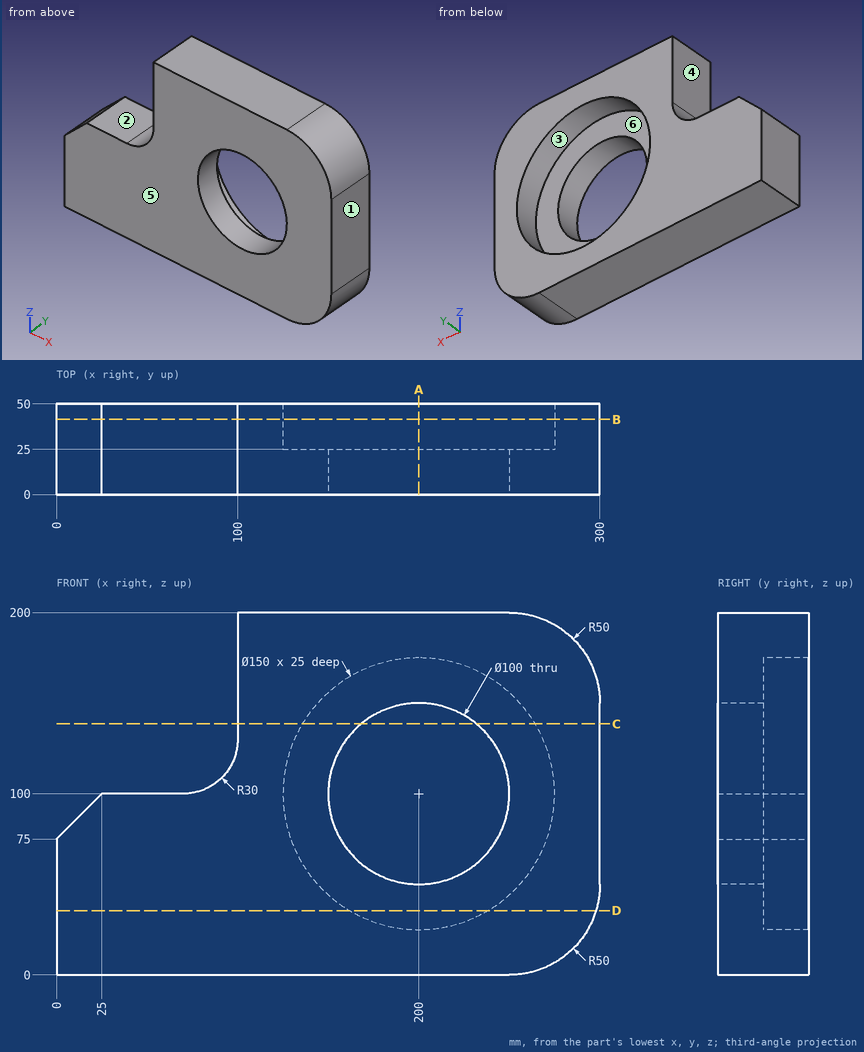
Geometry check sheet. Reference: drawing and pictorial views, mm from the part's lowest x, y, z. A direction names the side the tool comes from. Round coordinates to 2 decimals unless told otherwise and drop trailing zeros. Loops run counter-clockwise (first coordinate to the right, second up) from the corner with the lowest first, then second, coordinate; pieces in that order, holes last. Notation, with made-up numbers: (79.25, 43) -> (122.25, 43) arc R25 cw to (122.25, 80) -> close; hole circle Ø3 at (40, -6.75). An arc over 180 degrees is marked (long way). Answer as a JSON object with one key per item and string values.
Q1. Scan lines: line 1 (Z direction, x = 200, y = 16.25); line 2 (Z direction, x = 200, y = 35.25); line 3 (Y direction, x = 196, z = 32). Record each from-to range of solid material in increasing order. Write a range as from..to.
Data:
{"line 1": "z = 0..50, 150..200", "line 2": "z = 0..25, 175..200", "line 3": "y = 0..25"}
Q2. Section check A-A (x = 200). Record the boundary of the cut face in (y, z).
Data:
{"outline": "(0, 0) -> (50, 0) -> (50, 25) -> (25, 25) -> (25, 50) -> (0, 50) -> close; (0, 150) -> (25, 150) -> (25, 175) -> (50, 175) -> (50, 200) -> (0, 200) -> close"}
Q3. Section check B-B (y = 41.5). Record the boundary of the cut face in (x, z).
Data:
{"outline": "(0, 0) -> (250, 0) arc R50 ccw to (300, 50) -> (300, 150) arc R50 ccw to (250, 200) -> (100, 200) -> (100, 130) arc R30 cw to (70, 100) -> (25, 100) -> (0, 75) -> close; hole circle Ø150 at (200, 100)"}
Q4. Section check D-D (z = 35.5). Record the boundary of the cut face in (x, y).
Data:
{"outline": "(0, 0) -> (297.85, 0) -> (297.85, 50) -> (238.27, 50) -> (238.27, 25) -> (161.73, 25) -> (161.73, 50) -> (0, 50) -> close"}
Q5. Access from +Z, -Z, +X, -X, +Y, -Y to the whole of each face (thin tool, end or side, straight path). Record for the marked faces 4, 5 and 6.
Data:
{"face 4": "+Z, -X, +Y, -Y", "face 5": "+Z, -Z, +X, -X, -Y", "face 6": "+Y"}
Q6. Section check C-C (z = 138.5). Record the boundary of the cut face in (x, y), then the cut area to 3 significant figures.
Data:
{"outline": "(100, 0) -> (168.1, 0) -> (168.1, 25) -> (135.64, 25) -> (135.64, 50) -> (100, 50) -> close; (231.9, 0) -> (300, 0) -> (300, 50) -> (264.36, 50) -> (264.36, 25) -> (231.9, 25) -> close", "area": "5,190 mm2"}
Q7. Draft check along X on the marked faces 1, 2 and 3. Enter one of: pulls with the +X half, pulls with the -X half, needs draft (parallel to the pull), parting line crosses it, or undercut.
Data:
{"face 1": "pulls with the +X half", "face 2": "needs draft", "face 3": "undercut"}
